CAD build for the part. Positions are in the model's coordinates, mm. Face numbers are marked on the shaded views. A direction names the side the tool comes from. Coordinates: 2 decimals unless noted, no trailing zeros. Loops run counter-clockwise (first coordinate to the right, second up) from the corner with the lowest first, then second, coordinate; pieces in that order, holes last. Notation, with made-up numbers: (25.5, 9) -> (37.5, 9) arc R20 cw to (37.5, 14) -> close; hole circle Ø8 at (32, -18). An arc over 180 degrees is marked (long way). Answer as CSV lines item,"result". Start each with the question number.
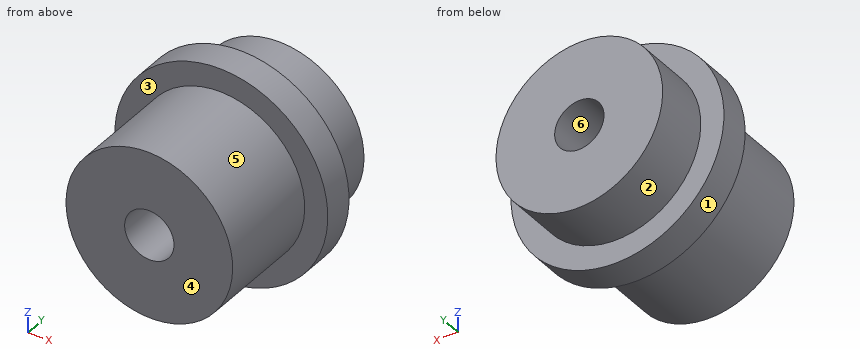
from build123d import *

# Parameters (mm, degrees)
BOSS_EXTRUDE1_DEPTH      = 11.43
BOSS_EXTRUDE1_DEPTH_BACK = 11.43
SKETCH1_R                = 17.145
SKETCH1_3_R              = 21.9075
SKETCH1_3_R_2            = 17.145
BOSS_EXTRUDE2_DEPTH      = 6.35
SKETCH1_4_R              = 17.145
BOSS_EXTRUDE3_DEPTH      = 27.94
CUT_EXTRUDE2_DEPTH       = 51.098642821
CUT_EXTRUDE2_DEPTH_BACK  = 51.098642821
SKETCH2_R                = 10.16
BOSS_EXTRUDE4_START      = -39.37
SKETCH3_R                = 10.16
SKETCH3_R_2              = 5.08
BOSS_EXTRUDE4_DEPTH      = 39.37


with BuildPart() as part:
    # Sketch1 → Boss-Extrude1 (new, two sides: drawn at the far end of the back side and taken through both)
    with BuildSketch(Plane(origin=(0, 0, 0), x_dir=(1, 0, 0), z_dir=(0, 1, 0)).offset(-BOSS_EXTRUDE1_DEPTH_BACK)):
        with Locations(Location((0, 0, 0), (0, 0, 270))):
            Circle(SKETCH1_R)
    extrude(amount=BOSS_EXTRUDE1_DEPTH + BOSS_EXTRUDE1_DEPTH_BACK)



with BuildPart() as body_2:
    # Sketch1<3> → Boss-Extrude2 (new body)
    with BuildSketch(Plane(origin=(0, 0, 0), x_dir=(1, 0, 0), z_dir=(0, 1, 0))):
        with Locations(Location((0, 0, 0), (0, 0, 270))):
            Circle(SKETCH1_3_R)
        with Locations(Location((0, 0, 0), (0, 0, 270))):
            Circle(SKETCH1_3_R_2, mode=Mode.SUBTRACT)
    extrude(amount=-BOSS_EXTRUDE2_DEPTH)


with BuildPart() as part_1:
    add(part.part)

    add(body_2.part)  # Boss-Extrude3 merges body 2
    # Sketch1<4> → Boss-Extrude3 (add)
    with BuildSketch(Plane(origin=(0, 0, 0), x_dir=(1, 0, 0), z_dir=(0, 1, 0))):
        with Locations(Location((0, 0, 0), (0, 0, 270))):
            Circle(SKETCH1_4_R)
    extrude(amount=-BOSS_EXTRUDE3_DEPTH)

    # Sketch2 → Cut-Extrude2 (cut, two sides: drawn at the far end of the back side and taken through both)
    with BuildSketch(Plane.XZ.offset(27.94).offset(-CUT_EXTRUDE2_DEPTH_BACK)):
        with Locations(Location((0, 0, 0), (0, 0, 270))):
            Circle(SKETCH2_R)
    extrude(amount=CUT_EXTRUDE2_DEPTH + CUT_EXTRUDE2_DEPTH_BACK, mode=Mode.SUBTRACT)

    # Sketch3 → Boss-Extrude4 (add)
    with BuildSketch(Plane(origin=(0, 11.43, 0), x_dir=(1, 0, 0), z_dir=(0, 1, 0)).offset(BOSS_EXTRUDE4_START)):
        Circle(SKETCH3_R)
        with Locations(Location((0, 0, 0), (0, 0, 270))):
            Circle(SKETCH3_R_2, mode=Mode.SUBTRACT)
    extrude(amount=BOSS_EXTRUDE4_DEPTH)


solid = part_1.part
Item 1: Saw through at D-D (x = 16.5). Write the cut outline in (y, z), plus the area to 3 significant figures.
Item 2: Flat gauge pins, fed straight in: pin 1 Ø6 at (y, z) = (-23.5, -12.5) entering from +X; pin 2 Ø2 at (x, y) = (-7.5, -6.5) entering from -Z; pin 3 Ø1 at (x, y) = (-13, -3.5) entering from +Z. Where does each tip first touch, or does it go through?
Item 3: Wall check: probe 1 along X at (y, z) = (-6, 0); probe 2 along X at (y, z) = (-12, 0) (3 decimals); probe 3 along Y at (x, z) = (6.5, 16.5). Give the ranges that are in metal, low to high.
Item 4: Saw through at C-C (y = -12.5). Write the cut outline in (x, z) (3 decimals), plus the area to 3 significant figures.
Item 5: Which spindle directions (+Z, -Z, +X, -X, +Y, -Y) get a long thin tool onto all of the face, cutting with end or side? Do the marked faces 1, 2 and 3. Say none if no direction does.
Item 6: Two-plate mould, pull along X, no slides. Class the marked faces 4, 5 and 6: pulls with the +X half, pulls with the -X half, needs draft (parallel to the pull), parting line crosses it, or undercut.
Geometry check:
1,outline,"(-27.94, -4.66) -> (-6.35, -4.66) -> (-6.35, -14.41) -> (0, -14.41) -> (0, -4.66) -> (11.43, -4.66) -> (11.43, 4.66) -> (0, 4.66) -> (0, 14.41) -> (-6.35, 14.41) -> (-6.35, 4.66) -> (-27.94, 4.66) -> close"
1,area,"491 mm2"
2,pin 1,"x = 14.27"
2,pin 2,"z = -20.92"
2,pin 3,"z = 17.99"
3,probe 1,"-21.91 to -5.08, 5.08 to 21.91"
3,probe 2,"-17.145 to -5.08, 5.08 to 17.145"
3,probe 3,"-6.35 to 0"
4,outline,"circle Ø34.29 at (0, 0); hole circle Ø10.16 at (0, 0)"
4,area,"842 mm2"
5,face 1,"+Y, -Y"
5,face 2,"+Y"
5,face 3,"-Y"
6,face 4,"needs draft"
6,face 5,"parting line crosses it"
6,face 6,"undercut"
